Build history of the part. All positions in model axes, mm. Face numbers are marked on the shaded views. A direction names the side the tool comes from. Round coordinates to 2 decimals unless told otherwise and drop trailing zeros. Write each loop counter-clockwise with the first axis right and the second up, starting at its lowest first coordinate (ties: lowest second). Pieces come first, ordered by that corner, then holes. Notation, with made-up numbers: (16.25, -27.5) -> (38.25, -27.5) arc R21 cw to (38.25, -13.5) -> close; hole circle Ø3 at (15.5, 7). An arc over 180 degrees is marked (long way). Answer in a Markdown table with one row per item.
```python
from build123d import *

# Parameters (mm, degrees)
SKETCH2_W           = 20
SKETCH2_H           = 30
SKETCH2_R           = 2
BOSS_EXTRUDE1_DEPTH = 1
SKETCH3_W           = 20
SKETCH3_H           = 1
BOSS_EXTRUDE2_DEPTH = 29
SKETCH4_R           = 2
CUT_EXTRUDE1_DEPTH  = 30


with BuildPart() as part:
    # Sketch2 → Boss-Extrude1 (new body)
    with BuildSketch(Plane(origin=(0, 0, 0), x_dir=(0, 0, -1), z_dir=(1, 0, 0))):
        with Locations((10, 15)):
            Rectangle(SKETCH2_W, SKETCH2_H)
        with Locations((10, 20)):
            Circle(SKETCH2_R, mode=Mode.SUBTRACT)
        with Locations((10, 10)):
            Circle(SKETCH2_R, mode=Mode.SUBTRACT)
    extrude(amount=BOSS_EXTRUDE1_DEPTH)

    # Sketch3 → Boss-Extrude2 (add)
    with BuildSketch(Plane(origin=(1, 0, 0), x_dir=(0, 0, -1), z_dir=(1, 0, 0))):
        with Locations((10, 29.5)):
            Rectangle(SKETCH3_W, SKETCH3_H)
    extrude(amount=BOSS_EXTRUDE2_DEPTH)

    # Sketch4 → Cut-Extrude1 (cut)
    with BuildSketch(Plane(origin=(0, 30, 0), x_dir=(1, 0, 0), z_dir=(0, 1, 0))):
        with Locations((15, 10)):
            Circle(SKETCH4_R)
    extrude(amount=-CUT_EXTRUDE1_DEPTH, mode=Mode.SUBTRACT)


solid = part.part
```
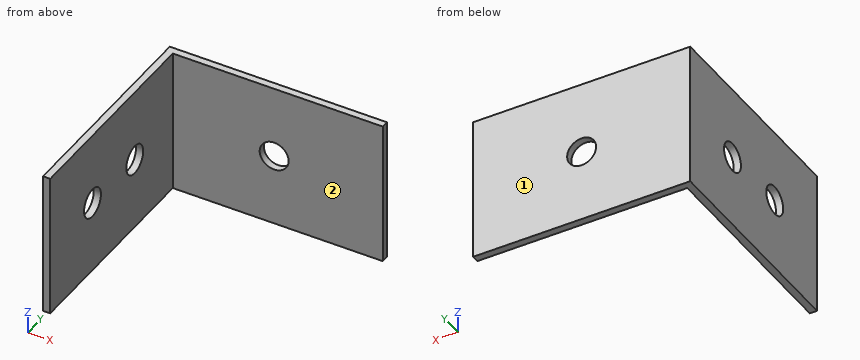
Q1. Saw through at A-A on z = -10. Write the cut outline in (x, y).
A:
| item | result |
|---|---|
| outline | (0, 0) -> (1, 0) -> (1, 8) -> (0, 8) -> close; (0, 12) -> (1, 12) -> (1, 18) -> (0, 18) -> close; (0, 22) -> (1, 22) -> (1, 29) -> (13, 29) -> (13, 30) -> (0, 30) -> close; (17, 29) -> (30, 29) -> (30, 30) -> (17, 30) -> close |
Q2. Saw through at B-B on y = 10. Write the cut outline in (x, z).
A:
| item | result |
|---|---|
| outline | (0, -20) -> (1, -20) -> (1, -12) -> (0, -12) -> close; (0, -8) -> (1, -8) -> (1, 0) -> (0, 0) -> close |
Q3. Wall check: line 1 (Y direction, x = 0.4, z = -10); line 2 (Z direction, x = 15, y = 29.7); line 3 (X direction, y = 29.3, z = -10). Give the ranges that are in metal, low to high. Write a range as [from, to].
A:
| item | result |
|---|---|
| line 1 | [0, 8], [12, 18], [22, 30] |
| line 2 | [-20, -12], [-8, 0] |
| line 3 | [0, 13], [17, 30] |
Q4. Saw through at D-D on x = 3. Write the cut outline in (y, z).
A:
| item | result |
|---|---|
| outline | (29, -20) -> (30, -20) -> (30, 0) -> (29, 0) -> close |
Q5. Saw through at C-C on z = -3. Write the cut outline in (x, y).
A:
| item | result |
|---|---|
| outline | (0, 0) -> (1, 0) -> (1, 29) -> (30, 29) -> (30, 30) -> (0, 30) -> close |
Q6. Which spindle directions (+Z, -Z, +X, -X, +Y, -Y) get a long thin tool onto all of the face, cutting with end or side? Do the marked faces 1 and 2. Say none if no direction does.
A:
| item | result |
|---|---|
| face 1 | +Z, -Z, +X, -X, +Y |
| face 2 | +Z, -Z, +X, -Y |
Q7. Drop flat-ended pins along their axis: P1, Ø4, axis at y = 8.5, z = -8, coming from the +X side; P2, Ø3, axis at x = 22, z = -4, coming from the -Y side. Give the stop position or say it passes through.
A:
| item | result |
|---|---|
| P1 | x = 1 |
| P2 | y = 29 |
